Check sheet for the drawn part. Datum: minimum x, y, z corner. Units: mm. A direction names the side the tool comes from. Coordinates: 2 decimals unless noted, no trailing zeros. Loops run counter-clockwise (first coordinate to the right, second up) from the corner with the lowest first, then second, coordinate; pieces in that order, holes last.
Q1. Material ranges on probe 1 along Z at (x, y) = (1.7, 5); probe 2 along Y at (x, z) = (3.2, 14.5); probe 3 along X at (y, z) = (6.75, 5.5), recorded low to high.
Q2. Go/stop test with flat-tipped pins: P1, Ø1, axis at x = 20, y = 5, coming from the +Z side; P2, Ø4.5, axis at y = 5, z = 14.5, coming from the +X side; P3, Ø6, axis at x = 9, y = 1.5, coming from the +Z side; P4, Ø6, axis at x = 5.5, z = 12.5, coming from the +Y side. Record where each tip stops, or that it passes through.
Q3. Sectioned sample at D-D (y = 1.25). Enter the section's corners in (x, z), then the cut area to 3 significant figures.
Q4. Sectioned sample at C-C (x = 2). Enter the section's corners in (y, z), then the cut area to 3 significant figures.
Q5. Sectioned sample at B-B (y = 5). Enter the section's corners in (x, z), then the cut area to 3 significant figures.
Q6. Sectioned sample at A-A (z = 14.5). Enter the section's corners in (x, y), then the cut area to 3 significant figures.
Q7. Mould release check, pull along X, two halves, no side actions. Record for the marked faces 1, 2, 3 and 4: +X half, -X half, draft (parallel to the pull), parting line (faces both ways), or undercut.
Q8. Access from +Z, -Z, +X, -X, +Y, -Y to the whole of each face (thin tool, end or side, straight path). Record for the marked faces 5 and 6.
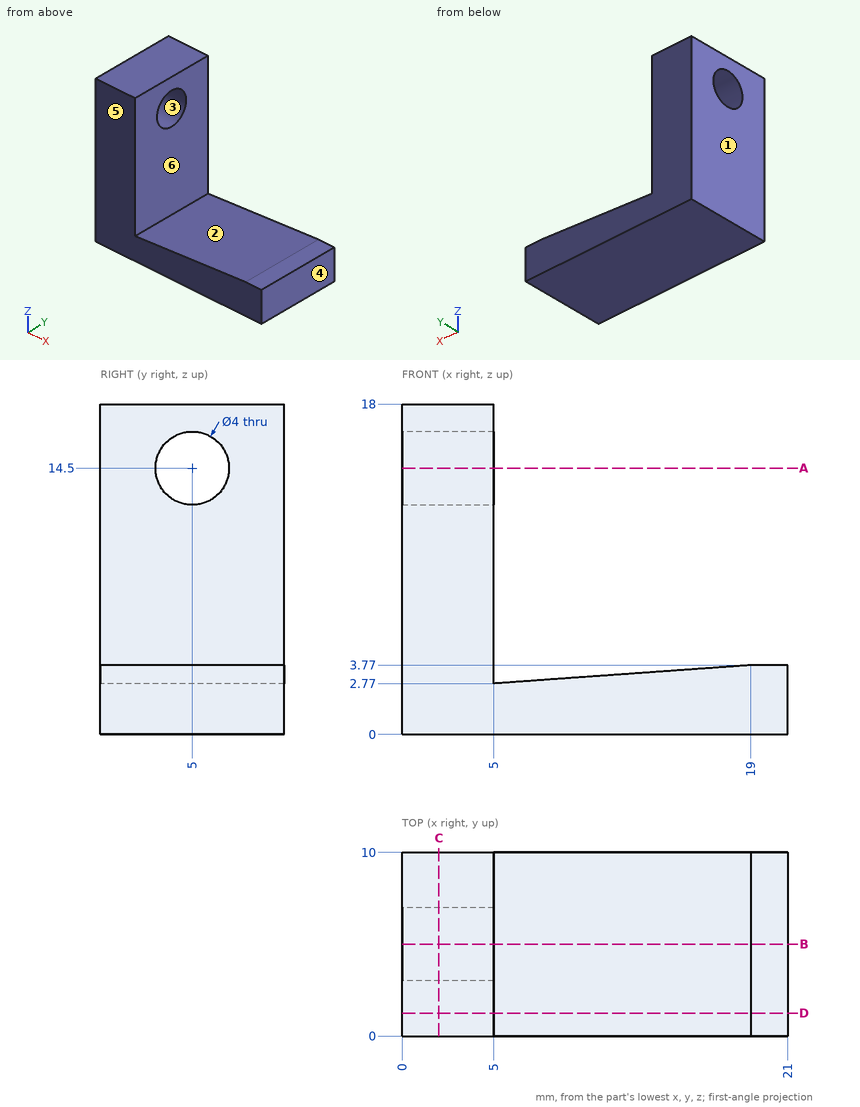
Geometry check:
1. probe 1: z = 0 to 12.5, 16.5 to 18
1. probe 2: y = 0 to 3, 7 to 10
1. probe 3: x = 0 to 5
2. P1: stops at z = 3.77
2. P2: stops at x = 5
2. P3: stops at z = 3.27
2. P4: stops at y = 10
3. outline: (0, 0) - (21, 0) - (21, 3.77) - (19, 3.77) - (5, 2.77) - (5, 18) - (0, 18) - close
3. area: 143 mm2
4. outline: (0, 0) - (10, 0) - (10, 18) - (0, 18) - close; hole circle Ø4 at (5, 14.5)
4. area: 167 mm2
5. outline: (0, 0) - (21, 0) - (21, 3.77) - (19, 3.77) - (5, 2.77) - (5, 12.5) - (0, 12.5) - close; (0, 16.5) - (5, 16.5) - (5, 18) - (0, 18) - close
5. area: 123 mm2
6. outline: (0, 0) - (5, 0) - (5, 3) - (0, 3) - close; (0, 7) - (5, 7) - (5, 10) - (0, 10) - close
6. area: 30.0 mm2
7. face 1: -X half
7. face 2: undercut
7. face 3: draft
7. face 4: +X half
8. face 5: +Z, -Z, +X, -X, -Y
8. face 6: +Z, +Y, -Y
